Source: CAD feature listing. Evaluate the final solid. Frame: model axes, mm. A direction names the side the tool comes from. Give positions to 0.01 mm unless a question says otherwise; leave off trailing zeros. Loops run counter-clockwise (first coordinate to the right, second up) from the corner with the lowest first, then second, coordinate; pieces in that order, holes last. Notation, with made-up numbers: (35, -14) -> (70, -14) arc R10 cw to (70, 0) -> close; hole circle Ø11 at (-13.75, -8.5). An arc over 180 degrees is marked (long way). Answer as a JSON object with one key per item and string values. Group by question number.
Autodesk Inventor part; units mm, degrees
ref_plane "YZ Plane" through (0, 0, 0) normal (1, 0, 0) x (0, 1, 0)
ref_plane "XZ Plane" through (0, 0, 0) normal (0, 1, 0) x (-1, 0, 0)
ref_plane "XY Plane" through (0, 0, 0) normal (0, 0, 1) x (1, 0, 0)
sketch "Sketch1" plane through (0, 0, 0) normal (0, 1, 0) x (-1, 0, 0)
  line L0 (16, 0) -> (0, 0)
  line L1 (0, 0) -> (0, -21)
  line L2 (0, -21) -> (6.6, -21)
  line L3 (6.6, -21) -> (6.6, -9)
  line L4 (6.6, -9) -> (33, -9)
  line L5 (33, -9) -> (33, -1)
  circle A0 centre (20, 0) radius 4
  line L6 (23.873, -1) -> (33, -1)
  line L7 (0, 0) -> (0, 21)
  line L8 (0, 21) -> (6.6, 21)
  line L9 (6.6, 21) -> (6.6, 9)
  line L10 (6.6, 9) -> (33, 9)
  line L11 (33, 9) -> (33, 1)
  circle A1 centre (20, 0) radius 4
  line L12 (23.873, 1) -> (33, 1)
  dimension "d0" = 6.6
  dimension "d1" = 21
  dimension "d2" = 1
  dimension "d3" = 9
  dimension "d4" = 8
  dimension "d5" = 33
  dimension "d19" = 20
extrude "Extrusion1" add sketch "Sketch1" along normal blind 14 contours A0 L6 L5 L4 L3 L2 L1 L0 | L0 L7 L8 L9 L10 L11 L12 A0
sketch "Sketch2" plane through (0, 0, 21) normal (1, 0, 0) x (0, 0, -1)
  circle A0 centre (38, 7) radius 2.5
  line L0 (21, 26.3461) -> (21, -5.4737) construction
  line L1 (0, 14) -> (42, 14)
  line L2 (42, 0) -> (42, 14)
  circle A1 centre (4, 7) radius 2.5
  point P0 (21, 0)
  point P1 (21, 14)
  point P2 (42, 7)
  dimension "d10" = 5
  dimension "d14" = 4
extrude "Extrusion2" cut sketch "Sketch2" against normal blind 14
sketch "Sketch3" plane through (-6.6, 0, -9) normal (0, 0, -1) x (-1, 0, 0)
  circle A0 centre (21.4, 7) radius 1.5
  line L0 (26.4, 0) -> (26.4, 14)
  point P0 (-6.6, 0)
  point P1 (26.4, 7)
  dimension "d15" = 3
  dimension "d16" = 5
extrude "Extrusion3" cut sketch "Sketch3" against normal up to surface (18 mm away)
equation "\"d17\" = d15"
properties part number "Shaft support - Stock"
(1) Mould query, pull axis X, two halves, no side actions, for faces 4 (the face through (-20, 7, -9)), 5 (the face through (-26.5, 7.07, 4.94)), 6 (the face through (-6.6, 7, -14)). Classes: pulls with the +X half, pulls with the -X half, needs draft (parallel to the pull), parting line crosses it, or undercut.
(2) Access query for faces 1 (the face through (-28, 5, 1)), 2 (the face through (-16, 7, 0)), 3 (the face through (-20, 7, 9)). Directions: +Z, -Z, +X, -X, +Y, -Y. A direction counts if a zero-diameter tool reaches every point of the face in a straight line with its end or side. Return the directions, or none.
(3) Section query B-B on x = -24.5. Return the cut outline in (y, z), plus the area to 3 significant figures.
(4) First-contact query: pin 1 (6 mm diameter, centred on y = 8.5, z = -16, fed in from -X); pin 2 (4.5 mm diameter, centred on x = -29, y = 5, fed in from -Z); pin 3 (1.5 mm diameter, centred on x = -10.5, y = 6, fed in from +Z). Flat tips, straight axial feed; report the tip coordinate or a pass-through.
(5) Section query D-D on z = -17. Return the cut outline in (x, y), plus the area to 3 significant figures.
(6) Section query A-A on z = -3. Return the cut outline in (x, y), plus the area to 3 significant figures.
(7) Material intervals for line 1 (Z direction, x = -26, y = 6.5); line 2 (Y direction, x = -28, z = -6.5); line 3 (X direction, y = 10.5, z = -15.5), sorted ascending. Write a range as from..to.
(8) Section query C-C on x = -28. Return the cut outline in (y, z).
Result:
{
 "1": {"face 4": "needs draft", "face 5": "undercut", "face 6": "pulls with the -X half"},
 "2": {"face 1": "-X, +Y, -Y", "face 2": "+Y, -Y", "face 3": "+Z, -X, +Y, -Y"},
 "3": {"outline": "(0, -9) -> (14, -9) -> (14, -1) -> (0, -1) -> close; (0, 1) -> (14, 1) -> (14, 9) -> (0, 9) -> close", "area": "224 mm²"},
 "4": {"pin 1": "x = -6.6", "pin 2": "z = -9", "pin 3": "z = 9"},
 "5": {"outline": "(-6.6, 0) -> (0, 0) -> (0, 4.5) -> (-6.6, 4.5) -> close; (-6.6, 9.5) -> (0, 9.5) -> (0, 14) -> (-6.6, 14) -> close", "area": "59.4 mm²"},
 "6": {"outline": "(-33, 0) -> (-22.65, 0) -> (-22.65, 14) -> (-33, 14) -> close; (-17.35, 0) -> (0, 0) -> (0, 14) -> (-17.35, 14) -> close; hole circle Ø3 at (-28, 7)", "area": "381 mm²"},
 "7": {"line 1": "-9..-1, 1..9", "line 2": "0..5.5, 8.5..14", "line 3": "-6.6..0"},
 "8": {"outline": "(0, -9) -> (5.5, -9) -> (5.5, -1) -> (0, -1) -> close; (0, 1) -> (5.5, 1) -> (5.5, 9) -> (0, 9) -> close; (8.5, -9) -> (14, -9) -> (14, -1) -> (8.5, -1) -> close; (8.5, 1) -> (14, 1) -> (14, 9) -> (8.5, 9) -> close"}
}
